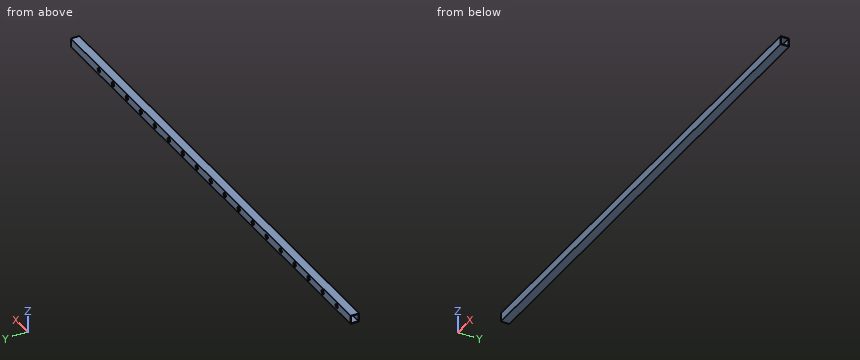
```python
from build123d import *

# Parameters (mm, degrees)
SKETCH1_W                      = 25.4
SKETCH1_H                      = 25.4
SKETCH1_W_2                    = 22.225
SKETCH1_H_2                    = 22.225
BOSS_EXTRUDE1_DEPTH            = 1524
F_1_2_0_5_DIAMETER_HOLE1_D     = 12.7
F_1_2_0_5_DIAMETER_HOLE1_DEPTH = 1.5875
LPATTERN1_COUNT                = 18
LPATTERN1_PITCH                = 76.2


with BuildPart() as part:
    # Sketch1 → Boss-Extrude1 (new body)
    with BuildSketch(Plane(origin=(0, 0, 0), x_dir=(0, 0, -1), z_dir=(1, 0, 0))):
        Rectangle(SKETCH1_W, SKETCH1_H)
        Rectangle(SKETCH1_W_2, SKETCH1_H_2, mode=Mode.SUBTRACT)
    extrude(amount=BOSS_EXTRUDE1_DEPTH)

    # 1/2 (0.5) Diameter Hole1
    with Locations(Plane(origin=(0, 12.7, 0), x_dir=(1, 0, 0), z_dir=(0, 1, 0))):
        with Locations((1371.6, 0)):
            f_1_2_0_5_diameter_hole1 = Hole(F_1_2_0_5_DIAMETER_HOLE1_D / 2, depth=F_1_2_0_5_DIAMETER_HOLE1_DEPTH)

    # LPattern1: 1/2 (0.5) Diameter Hole1 ×18
    with Locations(*[(-i * LPATTERN1_PITCH, 0, 0) for i in range(1, LPATTERN1_COUNT)]):
        add(f_1_2_0_5_diameter_hole1, mode=Mode.SUBTRACT)


solid = part.part
```
Geometry check sheet. Reference: the model listing, model coordinates, mm. Give positions to 0.01 mm unless a question says otherwise; leave off trailing zeros. Loops run counter-clockwise (first coordinate to the right, second up) from the corner with the lowest first, then second, coordinate; pieces in that order, holes last. Notation, with made-up numbers: M 16,7.5 L 70,7.5 A22 ccw 70,16.5 Z; hole C 67,12.25 d6. An arc over 180 degrees is marked long. Answer as CSV lines item,"result".
Item 1: Material ranges on line 1 (Z direction, x = 798.5, y = 3); line 2 (Z direction, x = 685.8, y = 12.1), recorded low to high.
Values:
line 1,"z = -12.7 to -11.11, 11.11 to 12.7"
line 2,"z = -12.7 to -6.35, 6.35 to 12.7"
Item 2: Cross-section at B-B on x = 1322. Record the cut outline in (y, z).
Values:
outline,"M -12.7,-12.7 L 12.7,-12.7 L 12.7,12.7 L -12.7,12.7 Z; hole M -11.11,-11.11 L 11.11,-11.11 L 11.11,11.11 L -11.11,11.11 Z"
Item 3: Depth check by flat-ended pin: P1, Ø7.5, axis at x = 1066.8, z = 0, coming from the +Y side. Enter the tip coordinate at first touch or a pass-through.
Values:
P1,"stops at y = -11.11"
Item 4: Cross-section at A-A on y = 6.75. Record the cut outline in (x, z), and give its area (3 significant figures).
Values:
outline,"M 0,-12.7 L 1524,-12.7 L 1524,-11.11 L 0,-11.11 Z; M 0,11.11 L 1524,11.11 L 1524,12.7 L 0,12.7 Z"
area,"4,840 mm²"
